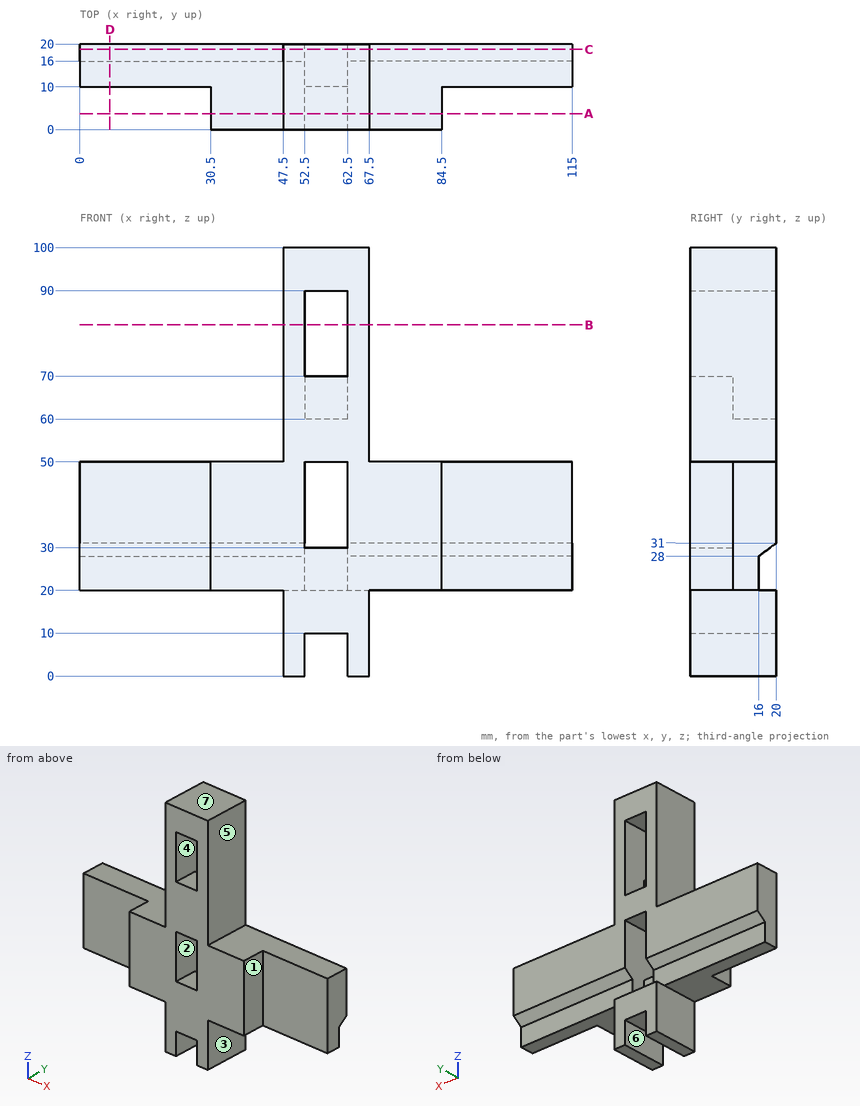
The figure shows three views and two pictorial views of one solid part (mm, origin at its lowest corner). Answer the questions. A direction names the side the tool comes from. Round coordinates to 2 decimals unless told otherwise and drop trailing zeros. Write each loop counter-clockwise with the first axis right and the second up, starting at its lowest first coordinate (ties: lowest second). Pieces come first, ordered by that corner, then holes. Notation, with made-up numbers: M 14,-9 L 52,-9 A24 ccw 52,17 Z; hole C 53,6 d1. An arc over 180 degrees is marked long. Use a Markdown table: item, result.
1) The part is cut by section A-A on y = 3.75. Give the vertices of the cut face in (x, z).
Taken from the geometry:
| item | result |
|---|---|
| outline | M 30.5,20 L 47.5,20 L 47.5,0 L 52.5,0 L 52.5,10 L 62.5,10 L 62.5,0 L 67.5,0 L 67.5,20 L 84.5,20 L 84.5,50 L 67.5,50 L 67.5,100 L 47.5,100 L 47.5,50 L 30.5,50 Z; hole M 52.5,30 L 62.5,30 L 62.5,50 L 52.5,50 Z; hole M 52.5,70 L 62.5,70 L 62.5,90 L 52.5,90 Z |
2) Flat-ended cylindrical pins translate along their axes: pin 1 (5 mm diameter, centred on x = 62, z = 89, fed in from +Y); pin 2 (6 mm diameter, centred on x = 25.5, y = 12.5, fed in from +Z); pin 3 (10 mm diameter, centred on y = 8.5, z = 85, fed in from -X); pin 4 (5 mm diameter, centred on x = 58.5, y = 5.5, fed in from -Z). Find the tip coordinate at first contact, or state that the pin passes through.
Taken from the geometry:
| item | result |
|---|---|
| pin 1 | stops at y = 20 |
| pin 2 | stops at z = 50 |
| pin 3 | stops at x = 47.5 |
| pin 4 | stops at z = 10 |
3) The part is cut by section B-B on z = 82. Give the vertices of the cut face in (x, y), plus the area to 3 significant figures.
Taken from the geometry:
| item | result |
|---|---|
| outline | M 47.5,0 L 52.5,0 L 52.5,20 L 47.5,20 Z; M 62.5,0 L 67.5,0 L 67.5,20 L 62.5,20 Z |
| area | 200 mm2 |
4) Consider line 1 (Z direction, x = 59, y = 18.5); line 2 (Z direction, x = 62, y = 7.5); line 3 (X direction, y = 8.75, z = 40). Determine where each line is inside the solid, lowest interval first. Write a range as [from, to].
Taken from the geometry:
| item | result |
|---|---|
| line 1 | z = [10, 20], [50, 60], [90, 100] |
| line 2 | z = [10, 30], [50, 70], [90, 100] |
| line 3 | x = [30.5, 52.5], [62.5, 84.5] |
5) The part is cut by section C-C on y = 18.75. Give the vertices of the cut face in (x, z).
Taken from the geometry:
| item | result |
|---|---|
| outline | M 0,30.06 L 52.5,30.06 L 52.5,50 L 62.5,50 L 62.5,30.06 L 115,30.06 L 115,50 L 67.5,50 L 67.5,100 L 47.5,100 L 47.5,50 L 0,50 Z; M 47.5,0 L 52.5,0 L 52.5,10 L 62.5,10 L 62.5,0 L 67.5,0 L 67.5,20 L 47.5,20 Z; hole M 52.5,60 L 62.5,60 L 62.5,90 L 52.5,90 Z |
6) Which of the six approach directions +Z, -Z, +X, -X, +Y, -Y give full straight-line access (tool end or side, diameter ignored) to the marked faces 1, 2 and 3?
Taken from the geometry:
| item | result |
|---|---|
| face 1 | +Z, -Z, +X, -Y |
| face 2 | +Y |
| face 3 | -Z, +X, +Y, -Y |
7) Determine the mould class of the marked faces 4, 5, 6 and 7 for opening direction X: pulls with the +X half, pulls with the -X half, needs draft (parallel to the pull), parting line crosses it, or undercut.
Taken from the geometry:
| item | result |
|---|---|
| face 4 | undercut |
| face 5 | pulls with the +X half |
| face 6 | undercut |
| face 7 | needs draft |
8) The part is cut by section D-D on x = 7. Give the vertices of the cut face in (y, z).
Taken from the geometry:
| item | result |
|---|---|
| outline | M 10,20 L 16,20 L 16,28 L 20,31 L 20,50 L 10,50 Z |
